```python
from build123d import *

# Parameters (mm, degrees)
SKETCH1_R           = 2
SKETCH1_W           = 5
SKETCH1_H           = 6
BOSS_EXTRUDE1_DEPTH = 9.5
CUT_EXTRUDE1_START  = 9.5
SKETCH1_6_R         = 2
SKETCH1_6_W         = 5
SKETCH1_6_H         = 6
CUT_EXTRUDE1_DEPTH  = 6.5
BOSS_EXTRUDE2_START = 3
SKETCH2_R           = 4
BOSS_EXTRUDE2_DEPTH = 3
BOSS_EXTRUDE3_START = 6
BOSS_EXTRUDE3_DEPTH = 3.5
CUT_EXTRUDE2_START  = 16.95
SKETCH3_R           = 2.25
CUT_EXTRUDE2_DEPTH  = 7
SKETCH5_R           = 1.6
CUT_EXTRUDE3_DEPTH  = 10
SKETCH6_W           = 17
SKETCH6_H           = 15
CUT_EXTRUDE4_DEPTH  = 1


with BuildPart() as part:
    # Sketch1 → Boss-Extrude1 (new body)
    with BuildSketch(Plane(origin=(0, 0, 0), x_dir=(0, 0, -1), z_dir=(1, 0, 0))):
        with BuildLine():
            Line((-12.5, -5), (-12.5, 20))
            Line((-12.5, 20), (12.5, 20))
            Line((12.5, 20), (12.5, -5))
            Line((12.5, -5), (3.003242416, -14.592070209))
            ThreePointArc((3.003242416, -14.592070209), (0, -15.95), (-3.003242416, -14.592070209))
            Line((-3.003242416, -14.592070209), (-12.5, -5))
        make_face()
        with Locations((0, -11.95)):
            Circle(SKETCH1_R, mode=Mode.SUBTRACT)
        with BuildLine():
            Line((-3.31662479, 6.95), (3.31662479, 6.95))
            ThreePointArc((3.31662479, 6.95), (6, 11.95), (3.31662479, 16.95))
            Line((3.31662479, 16.95), (-3.31662479, 16.95))
            ThreePointArc((-3.31662479, 16.95), (-6, 11.95), (-3.31662479, 6.95))
        make_face(mode=Mode.SUBTRACT)
        Rectangle(SKETCH1_W, SKETCH1_H, mode=Mode.SUBTRACT)
    extrude(amount=BOSS_EXTRUDE1_DEPTH)

    # Sketch1<6> → Cut-Extrude1 (cut)
    with BuildSketch(Plane(origin=(0, 0, 0), x_dir=(0, 0, -1), z_dir=(1, 0, 0)).offset(CUT_EXTRUDE1_START)):
        with BuildLine():
            ThreePointArc((-8.865865393, -4.625627615), (-9.724278097, -5.810910858), (-10.425207588, -7.09561572))
            Line((-10.425207588, -7.09561572), (-3.003242416, -14.592070209))
            ThreePointArc((-3.003242416, -14.592070209), (0, -15.95), (3.003242416, -14.592070209))
            Line((3.003242416, -14.592070209), (10.425207588, -7.09561572))
            ThreePointArc((10.425207588, -7.09561572), (9.724278097, -5.810910858), (8.865865393, -4.625627615))
            ThreePointArc((8.865865393, -4.625627615), (9.731180291, 2.303069722), (5.85199823, 8.108891213))
            ThreePointArc((5.85199823, 8.108891213), (0, 18.95), (-5.85199823, 8.108891213))
            ThreePointArc((-5.85199823, 8.108891213), (-9.731180291, 2.303069722), (-8.865865393, -4.625627615))
        make_face()
        with Locations((0, -11.95)):
            Circle(SKETCH1_6_R, mode=Mode.SUBTRACT)
        Rectangle(SKETCH1_6_W, SKETCH1_6_H, mode=Mode.SUBTRACT)
        with BuildLine():
            Line((3.31662479, 6.95), (-3.31662479, 6.95))
            ThreePointArc((-3.31662479, 6.95), (-6, 11.95), (-3.31662479, 16.95))
            Line((-3.31662479, 16.95), (3.31662479, 16.95))
            ThreePointArc((3.31662479, 16.95), (6, 11.95), (3.31662479, 6.95))
        make_face(mode=Mode.SUBTRACT)
    extrude(amount=-CUT_EXTRUDE1_DEPTH, mode=Mode.SUBTRACT)

    # Sketch2 → Boss-Extrude2 (add)
    with BuildSketch(Plane(origin=(0, 0, 0), x_dir=(0, 0, -1), z_dir=(1, 0, 0)).offset(BOSS_EXTRUDE2_START)):
        with BuildLine():
            Line((6.975447566, 11.364225941), (5.978955057, -0.50209205))
            ThreePointArc((5.978955057, -0.50209205), (0.004288423, -5.999998467), (-5.978231221, -0.510638298))
            Line((-5.978231221, -0.510638298), (-6.954880764, 11.156505474))
            ThreePointArc((-6.954880764, 11.156505474), (-0.104368082, 18.949221907), (6.975447566, 11.364225941))
        make_face()
        Circle(SKETCH2_R, mode=Mode.SUBTRACT)
        with BuildLine():
            Line((-3.31662479, 16.95), (3.31662479, 16.95))
            ThreePointArc((3.31662479, 16.95), (6, 11.95), (3.31662479, 6.95))
            Line((3.31662479, 6.95), (-3.31662479, 6.95))
            ThreePointArc((-3.31662479, 6.95), (-6, 11.95), (-3.31662479, 16.95))
        make_face(mode=Mode.SUBTRACT)
    extrude(amount=BOSS_EXTRUDE2_DEPTH)

    # Sketch4 → Boss-Extrude3 (add)
    with BuildSketch(Plane(origin=(0, 0, 0), x_dir=(0, 0, -1), z_dir=(1, 0, 0)).offset(BOSS_EXTRUDE3_START)):
        with BuildLine():
            Line((-4.898979486, 16.95), (4.898979486, 16.95))
            ThreePointArc((4.898979486, 16.95), (0, 18.95), (-4.898979486, 16.95))
        make_face()
    extrude(amount=BOSS_EXTRUDE3_DEPTH)

    # Sketch3 → Cut-Extrude2 (cut)
    with BuildSketch(Plane(origin=(0, 0, 0), x_dir=(1, 0, 0), z_dir=(0, 1, 0)).offset(CUT_EXTRUDE2_START)):
        with Locations((9.5, 0)):
            Circle(SKETCH3_R)
    extrude(amount=CUT_EXTRUDE2_DEPTH, mode=Mode.SUBTRACT)

    # Sketch5 → Cut-Extrude3 (cut)
    with BuildSketch(Plane(origin=(0, 0, 0), x_dir=(0, 0, -1), z_dir=(1, 0, 0))):
        with Locations((8.5, 17.5)):
            Circle(SKETCH5_R)
        with Locations((-8.5, 17.5)):
            Circle(SKETCH5_R)
        with Locations((9, 9)):
            Circle(SKETCH5_R)
        with Locations((-9.5, 9)):
            Circle(SKETCH5_R)
    extrude(amount=CUT_EXTRUDE3_DEPTH, mode=Mode.SUBTRACT)

    # Sketch6 → Cut-Extrude4 (cut)
    with BuildSketch(Plane(origin=(0, 0, 0), x_dir=(0, 0, -1), z_dir=(1, 0, 0))):
        Rectangle(SKETCH6_W, SKETCH6_H)
    extrude(amount=CUT_EXTRUDE4_DEPTH, mode=Mode.SUBTRACT)


solid = part.part
```
For this review, take the finished solid that the model builds, in its own axes (mm). A direction names the side the tool comes from. Coordinates: 2 decimals unless noted, no trailing zeros. Order: outer loops, then holes, each group sorted by start corner. A loop starts at its lowest first (then second) coordinate and runs counter-clockwise, first axis right, second up. Notation, with made-up numbers: (83.25, 50.5) -> (119.25, 50.5) arc R22 cw to (119.25, 74.5) -> close; hole circle Ø9 at (-38.75, 10.5). An arc over 180 degrees is marked (long way). Use CSV: the item, a comma, the result in double quotes. Start each with the question number.
Item 1: Wall thickness on probe 1 along Y at (x, z) = (4.6, 0); probe 2 along Z at (x, y) = (5.5, 17.5); probe 3 along Z at (x, y) = (5.75, -1.5): over which ranges is each line inside the solid? List them lowest first.
Item 2: We need section D-D, the plane y = -11.95. Give the boundary of the cut face in (x, z), then the cut area to 3 significant figures.
Item 3: For faces 5 (the face through (3, 0, -3)), 6 (the face through (6.296, -5.828, -9.735)), 7 (the face through (2, 0, 2.5)), 8 (the face through (0.5, -0.1, -8.5)), list the 3-axis set-ups (+Z, -Z, +X, -X, +Y, -Y) from which the entire face can be reached by the end or side of a thin tool; tool diameter is ignored.
Item 4: We need section C-C, the plane z = 0. Give the boundary of the cut face in (x, y).
Item 5: We need section A-A, the plane y = 17.5. Give the boundary of the cut face in (x, z), then the cut area to 3 significant figures.
Item 6: Draft analysis for pull direction Z (two halves, no side actions). For faces 1 (the face through (2.57, -8.8, 8.74)), 2 (the face through (5, 8, -12.5)), 3 (the face through (4.684, 19.086, 8.708)), 4 (the face through (6.296, 2.4, 9.708)), state which applies: pulls with the +Z half, pulls with the -Z half, needs draft (parallel to the pull), parting line crosses it, or undercut.
Item 7: We need section B-B, the plane x = 8. Give the boundary of the cut face in (y, z), then the cut area to 3 significant figures.
Item 8: Insertion check: pin 1 (3 mm diameter, centred on y = 9, z = -9, fed in from +X); pin 2 (3 mm diameter, centred on y = -7, z = -3, fed in from +X); pin 3 (10.5 mm diameter, centred on y = 0, z = 0, fed in from -X); pin 4 (3 mm diameter, centred on y = -11, z = -6.5, fed in from -X). Each pin has a flat end and moves straight along its axis. Give the tip position at first contact, or say it passes through.
Derived:
1,probe 1,"y = -6 to -4, 4 to 6.95, 16.95 to 20"
1,probe 2,"z = -12.5 to -10.1, -6.9 to 6.9, 10.1 to 12.5"
1,probe 3,"z = -12.5 to -9.89, -5.81 to -3.71, 3.71 to 5.81, 9.89 to 12.5"
2,outline,"(0, -5.62) -> (3, -5.62) -> (3, -2) -> (0, -2) -> close; (0, 2) -> (3, 2) -> (3, 5.62) -> (0, 5.62) -> close"
2,area,"21.7 mm^2"
3,face 5,"+X"
3,face 6,"+X, -Y"
3,face 7,"+X, -X"
3,face 8,"-X"
4,outline,"(0, -15.95) -> (3, -15.95) -> (3, -13.95) -> (0, -13.95) -> close; (0, -9.95) -> (3, -9.95) -> (3, -6) -> (6, -6) -> (6, -4) -> (3, -4) -> (3, -3) -> (1, -3) -> (1, -7.5) -> (0, -7.5) -> close; (0, 16.95) -> (7.25, 16.95) -> (7.25, 20) -> (0, 20) -> close; (1, 3) -> (3, 3) -> (3, 4) -> (6, 4) -> (6, 6.95) -> (1, 6.95) -> close"
5,outline,"(0, -12.5) -> (9.5, -12.5) -> (9.5, -10.1) -> (0, -10.1) -> close; (0, -6.9) -> (9.5, -6.9) -> (9.5, -2.25) arc R2.25 cw to (9.5, 2.25) -> (9.5, 6.9) -> (0, 6.9) -> close; (0, 10.1) -> (9.5, 10.1) -> (9.5, 12.5) -> (0, 12.5) -> close"
5,area,"169 mm^2"
6,face 1,"pulls with the +Z half"
6,face 2,"pulls with the -Z half"
6,face 3,"undercut"
6,face 4,"undercut"
7,outline,"(-7.1, -10.43) -> (-5, -12.5) -> (20, -12.5) -> (20, -1.68) -> (16.95, -1.68) -> (16.95, -4.9) arc R7 cw to (8.11, -5.85) arc R10 cw to (-4.63, -8.87) arc R11.5 cw to start; (-7.1, 10.43) arc R11.5 cw to (-4.63, 8.87) arc R10 cw to (8.11, 5.85) arc R7 cw to (16.95, 4.9) -> (16.95, 1.68) -> (20, 1.68) -> (20, 12.5) -> (-5, 12.5) -> close; hole circle Ø3.2 at (9, -9); hole circle Ø3.2 at (9, 9.5); hole circle Ø3.2 at (17.5, -8.5); hole circle Ø3.2 at (17.5, 8.5)"
7,area,"237 mm^2"
8,pin 1,"passes through"
8,pin 2,"stops at x = 3"
8,pin 3,"stops at x = 1"
8,pin 4,"stops at x = 0"
